The listing builds one solid part. Answer for the finished solid, in the listing's coordinates (mm). Face numbers are marked on the shaded views. A direction names the side the tool comes from. Round coordinates to 2 decimals unless told otherwise and drop trailing zeros. Write each loop counter-clockwise with the first axis right and the second up, starting at its lowest first coordinate (ties: lowest second). Pieces come first, ordered by that corner, then holes.
Autodesk Inventor part; units mm, degrees
ref_plane "YZ Plane" through (0, 0, 0) normal (1, 0, 0) x (0, 1, 0)
ref_plane "XZ Plane" through (0, 0, 0) normal (0, 1, 0) x (-1, 0, 0)
ref_plane "XY Plane" through (0, 0, 0) normal (0, 0, 1) x (1, 0, 0)
sketch "Boceto1" plane through (0, 0, 0) normal (0, 1, 0) x (-1, 0, 0)
  circle A0 centre (0, 0) radius 6.05
  circle A1 centre (0, 0) radius 6.85
  dimension "d0" = 12.1
  dimension "d1" = 0.8
extrude "Extrusión1" add sketch "Boceto1" along normal mid plane 6.35
sketch "Boceto2" plane through (0, 3.175, 0) normal (0, 1, 0) x (1, 0, 0)
  circle A0 centre (0, 0) radius 6.05
  circle A1 centre (0, 0) radius 8.75
  dimension "d4" = 17.5
extrude "Extrusión2" add sketch "Boceto2" along normal blind 1.12
sketch "Boceto3" plane through (0, -3.175, 0) normal (0, -1, 0) x (1, 0, 0)
  circle A0 centre (0, 0) radius 6.05
  circle A1 centre (0, 0) radius 8.75
  circle A2 centre (0, 0) radius 8.75
extrude "Extrusión3" add sketch "Boceto3" along normal blind 1.12
sketch "Boceto4" plane through (0, 4.295, 0) normal (0, 1, 0) x (1, 0, 0)
  circle A0 centre (0, 0) radius 6.05
  circle A1 centre (0, 0) radius 4.5
  dimension "d14" = 9
extrude "Extrusión4" add sketch "Boceto4" against normal blind 2.295
sketch "Boceto6" plane through (0, 3.175, 0) normal (0, -1, 0) x (1, 0, 0)
  circle A0 centre (0, 0) radius 6.85
  circle A1 centre (0, 0) radius 8.53
  circle A2 centre (0, 0) radius 7.78
  dimension "d17" = 1.68
  dimension "d18" = 0.75
fillet "Empalme1" radius 1 1 edges at (-6.05, -4.295, 0)
sketch "Boceto7" plane through (0, 4.295, 0) normal (0, 1, 0) x (1, 0, 0)
  circle A0 centre (0, 0) radius 8.75
  circle A1 centre (0, 0) radius 6.85
  circle A2 centre (0, 0) radius 6.85
extrude "Extrusión6" cut sketch "Boceto7" against normal up to surface (7.47 mm away)
sketch "Boceto5" plane through (0, -4.295, 0) normal (0, -1, 0) x (1, 0, 0)
  circle A0 centre (0, 0) radius 8.75
  circle A1 centre (0, 0) radius 6.85
properties part number "Idle pulley"
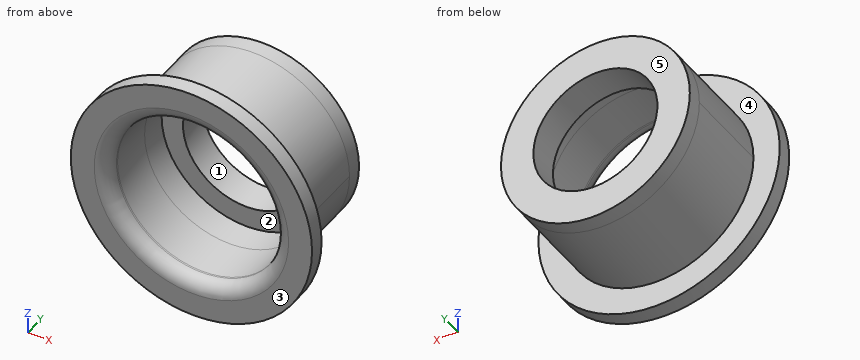
1. A tool of negligible diameter and unlimited length cuts with its end or side. For the marked faces 4 and 5, from which of +Z, -Z, +X, -X, +Y, -Y can it reach the whole face along a straight path? Write none if from no direction.
Geometry says:
face 4: +Y
face 5: +Z, -Z, +X, -X, +Y
2. Given pin 1 (3 mm diameter, centred on x = -2.5, y = -1, fed in from +Z); pin 2 (1 mm diameter, centred on x = 6, y = -1.5, fed in from -Z); pin 3 (5 mm diameter, centred on y = 3, z = 6, fed in from +X); pin 4 (7.5 mm diameter, centred on x = 0, z = 0, fed in from -Y), each flat-ended and moving along its own axis, determine where each tip first touches the part or whether it passes through.
Geometry says:
pin 1: stops at z = 6.78
pin 2: stops at z = -4.08
pin 3: stops at x = 5.89
pin 4: passes through
3. Section B-B on y = 2.75 is taken. Determine the outline of the cut face in (x, z).
Geometry says:
outline: circle Ø13.7 at (0, 0); hole circle Ø9 at (0, 0)
4. For a pull along X with two mould halves and no side action, classify the marked faces 1, 2 and 3 as released by +X, released by -X, zero draft, split by the parting line, or undercut.
Geometry says:
face 1: undercut
face 2: undercut
face 3: zero draft
5. Section A-A on x = 0 is taken. Determine the outline of the cut face in (y, z) (3 decimals).
Geometry says:
outline: (-4.295, -8.75) - (-3.175, -8.75) - (-3.175, -6.85) - (4.295, -6.85) - (4.295, -4.5) - (2, -4.5) - (2, -6.05) - (-3.295, -6.05) arc R1 ccw to (-4.295, -7.05) - close; (-4.295, 7.05) arc R1 ccw to (-3.295, 6.05) - (2, 6.05) - (2, 4.5) - (4.295, 4.5) - (4.295, 6.85) - (-3.175, 6.85) - (-3.175, 8.75) - (-4.295, 8.75) - close
6. Straight lines are drawn through the part: line 1 along Z through (x, y) = (0, 1.25); line 2 along X through (y, z) = (3.05, 0). For each, find the intervals that lie inside material, in ascending order.
Geometry says:
line 1: z = -6.85 to -6.05, 6.05 to 6.85
line 2: x = -6.85 to -4.5, 4.5 to 6.85
7. Section D-D on z = 7.75 is taken. Determine the outline of the cut face in (x, y) (3 decimals).
Geometry says:
outline: (-4.062, -4.295) - (4.062, -4.295) - (4.062, -3.175) - (-4.062, -3.175) - close
8. Section C-C on y = 1 is taken. Determine the outline of the cut face in (x, z).
Geometry says:
outline: circle Ø13.7 at (0, 0); hole circle Ø12.1 at (0, 0)
